Autodesk Inventor part; units mm, degrees
ref_plane "YZ Plane" through (0, 0, 0) normal (1, 0, 0) x (0, 1, 0)
ref_plane "XZ Plane" through (0, 0, 0) normal (0, 1, 0) x (-1, 0, 0)
ref_plane "XY Plane" through (0, 0, 0) normal (0, 0, 1) x (1, 0, 0)
sketch "Sketch1" plane through (0, 0, 0) normal (0, 0, 1) x (1, 0, 0)
  line L0 (-5.55, -4.05) -> (5.55, -4.05)
  line L1 (5.55, -4.05) -> (5.55, 4.05)
  line L2 (5.55, 4.05) -> (-5.55, 4.05)
  line L3 (-5.55, 4.05) -> (-5.55, -4.05)
  line L4 (-5.55, -4.05) -> (5.55, 4.05) construction
  line L5 (5.55, -4.05) -> (-5.55, 4.05) construction
  line L6 (-4.75, 0.55) -> (4.75, 0.55)
  line L7 (4.75, 0.55) -> (4.75, 7.55)
  line L8 (4.75, 7.55) -> (-4.75, 7.55)
  line L9 (-4.75, 7.55) -> (-4.75, 0.55)
  line L10 (-4.75, 0.55) -> (4.75, 7.55) construction
  line L11 (4.75, 0.55) -> (-4.75, 7.55) construction
  line L12 (5.85, -4.55) -> (-7.55, -4.55)
  line L13 (-7.55, -4.55) -> (-7.55, 4.55)
  line L14 (-7.55, 4.55) -> (5.85, 4.55)
  line L15 (5.85, 4.55) -> (5.85, -4.55)
  line L16 (-17.05, -2.45) -> (-9.05, -2.45)
  line L17 (-9.05, -2.45) -> (-9.05, 2.55)
  line L18 (-9.05, 2.55) -> (-17.05, 2.55)
  line L19 (-17.05, 2.55) -> (-17.05, -2.45)
  line L20 (-17.05, -2.45) -> (-9.05, 2.55) construction
  line L21 (-9.05, -2.45) -> (-17.05, 2.55) construction
  line L22 (-18.55, -3.45) -> (-7.55, -3.45)
  line L23 (-7.55, -3.45) -> (-7.55, 3.55)
  line L24 (-7.55, 3.55) -> (-18.55, 3.55)
  line L25 (-18.55, 3.55) -> (-18.55, -3.45)
  line L26 (-18.55, -3.45) -> (-7.55, 3.55) construction
  line L27 (-7.55, -3.45) -> (-18.55, 3.55) construction
  point P0 (0, 0)
  point P1 (0, 4.05)
  point P2 (4.75, 4.05)
  point P3 (-4.75, 4.05)
  point P4 (-13.05, 0.05)
  point P5 (-7.55, -3.45)
  dimension "d0" = 11.1
  dimension "d1" = 8.1
  dimension "d2" = 9.5
  dimension "d3" = 4.6
  dimension "d8" = 0.5
  dimension "d9" = 2
  dimension "d10" = 0.5
  dimension "d11" = 0.3
  dimension "d14" = 8
  dimension "d15" = 5
  dimension "d16" = 1.5
  dimension "d17" = 22.6
  dimension "d18" = 7
extrude "Extrusion1" add sketch "Sketch1" along normal blind 2.7 contours L3 L2 L9 L6 L7 L1 L0
fillet "Fillet1" radius 0.5 4 edges at (5.55, 4.05, 1.35) (5.55, -4.05, 1.35) (-5.55, -4.05, 1.35) (-5.55, 4.05, 1.35)
fillet "Fillet2" radius 0.3 2 edges at (-4.75, 0.55, 1.35) (4.75, 0.55, 1.35)
extrude "Extrusion2" add sketch "Sketch1" against normal blind 1 contours L3 L2 L9 L6 L7 L1 L0 | L0 L1 L2 L7 L14 L15 L12 L13 L9 L3 | L9 L14 L7 L2
extrude "Extrusion3" add sketch "Sketch1" against normal up to surface (1 mm away) contours L13 L22 L25 L24 | L19 L18 L17 L16
extrude "Extrusion4" add sketch "Sketch1" along normal up to surface (2.7 mm away) contours L19 L18 L17 L16
chamfer "Chamfer1" distance 0.8 angle 45 2 edges at (-9.05, 2.55, 1.35) (-17.05, 2.55, 1.35)
fillet "Fillet3" radius 0.5 6 edges at (-9.85, 2.55, 1.35) (-9.05, 1.75, 1.35) (-9.05, -2.45, 1.35) (-16.25, 2.55, 1.35) (-17.05, 1.75, 1.35) (-17.05, -2.45, 1.35)
properties part number "firewire-02"
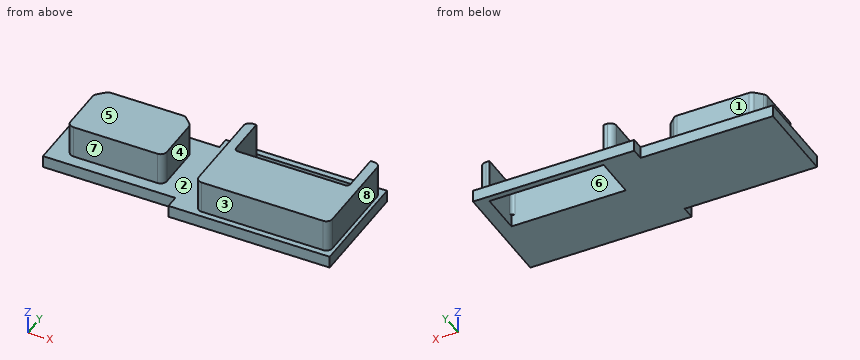
CAD build for the part. Positions are in the model's coordinates, mm. Face numbers are marked on the shaded views. A direction names the side the tool comes from. Give positions to 0.01 mm unless a question says otherwise; leave off trailing zeros. Write each loop counter-clockwise with the first axis right and the second up, starting at its lowest first coordinate (ties: lowest second). Pieces come first, ordered by that corner, then holes. Notation, with made-up numbers: (41.5, 89.5) - (56.5, 89.5) arc R21 cw to (56.5, 96.5) - close; hole circle Ø8 at (81.25, 5.5). An arc over 180 degrees is marked (long way). Answer as CSV lines item,"result".
Q1. Band-saw the part on D-D (x = -12). Give the cut face in (y, z).
Result set:
outline,"(-3.45, -1) - (3.55, -1) - (3.55, 0) - (2.55, 0) - (2.55, 2.7) - (-2.45, 2.7) - (-2.45, 0) - (-3.45, 0) - close"
Q2. Drill centre lines: line 1 (X direction, y = 0.25, z = 1.25); line 2 (X direction, y = 3, z = 1.6); line 3 (X direction, y = 2, z = 0.05). Where is each one in solid material? Low to high. Write a range as from..to.
Result set:
line 1,"-17.05..-9.05, -5.55..5.55"
line 2,"-5.55..-4.75, 4.75..5.55"
line 3,"-16.8..-9.3, -5.55..-4.75, 4.75..5.55"
Q3. Band-saw the part on C-C (z = 2.3). Give the cut face in (x, y).
Result set:
outline,"(-17.05, -1.95) arc R0.5 ccw to (-16.55, -2.45) - (-9.55, -2.45) arc R0.5 ccw to (-9.05, -1.95) - (-9.05, 1.54) arc R0.5 ccw to (-9.2, 1.9) - (-9.7, 2.4) arc R0.5 ccw to (-10.06, 2.55) - (-16.04, 2.55) arc R0.5 ccw to (-16.4, 2.4) - (-16.9, 1.9) arc R0.5 ccw to (-17.05, 1.54) - close; (-5.55, -3.55) arc R0.5 ccw to (-5.05, -4.05) - (5.05, -4.05) arc R0.5 ccw to (5.55, -3.55) - (5.55, 3.55) arc R0.5 ccw to (5.05, 4.05) - (4.75, 4.05) - (4.75, 0.85) arc R0.3 cw to (4.45, 0.55) - (-4.45, 0.55) arc R0.3 cw to (-4.75, 0.85) - (-4.75, 4.05) - (-5.05, 4.05) arc R0.5 ccw to (-5.55, 3.55) - close"
Q4. Flat gauge pins, fed straight in: pin 1 Ø0.8 at (x, z) = (-14.5, 1) entering from -Y; pin 2 Ø3 at (x, y) = (-2, 3.5) entering from +Z; pin 3 Ø0.8 at (x, z) = (-14, -0.5) entering from -Y. Where does each tip first touch, or does it go through?
Result set:
pin 1,"y = -2.45"
pin 2,"z = 0"
pin 3,"y = -3.45"
Q5. 3-axis set-ups, long thin cutter, end or side, ignore diameter. For the marked faces 1, 2, 3, 4 and 5: which of +Z, -Z, +X, -X, +Y, -Y reach the whole face in a straight line?
Result set:
face 1,"+Z, -X, +Y"
face 2,"+Z"
face 3,"+Z, +X, -X, -Y"
face 4,"+Z, +Y, -Y"
face 5,"+Z, +X, -X, +Y, -Y"
Q6. Pull direction X, two halves, no side cores. Call the marked faces 6, 7 and 8: released by +X, released by -X, zero draft, split by the parting line, or undercut.
Result set:
face 6,"undercut"
face 7,"zero draft"
face 8,"released by +X"
Q7. Band-saw the part on B-B (y = -0.5). Give the cut face in (x, z), and give its area (3 significant figures).
Result set:
outline,"(-18.55, -1) - (5.85, -1) - (5.85, 0) - (5.55, 0) - (5.55, 2.7) - (-5.55, 2.7) - (-5.55, 0) - (-9.05, 0) - (-9.05, 2.7) - (-17.05, 2.7) - (-17.05, 0) - (-18.55, 0) - close"
area,"76.0 mm²"
Q8. Band-saw the part on A-A (x = -1). Give the cut face in (y, z), and give its area (3 significant figures).
Result set:
outline,"(-4.55, -1) - (0.55, -1) - (0.55, 2.7) - (-4.05, 2.7) - (-4.05, 0) - (-4.55, 0) - close; (4.05, -1) - (4.55, -1) - (4.55, 0) - (4.05, 0) - close"
area,"18.0 mm²"
